Build history of the part. All positions in model axes, mm. A direction names the side the tool comes from. Coordinates: 2 decimals unless noted, no trailing zeros. Order: outer loops, then holes, each group sorted by start corner. A loop starts at its lowest first (then second) coordinate and runs counter-clockwise, first axis right, second up. Notation, with made-up numbers: M 59,-1 L 95,-1 A22 ccw 95,25 Z; hole C 84,-1 d4. An arc over 180 degrees is marked long. Write item = value, one per line. Start each with the question number.
Q1. Pin check, flat tip, straight feed: P1, Ø0.6, axis at y = 0, z = -0.5, coming from the -X side. Stop position of the tip, or through.
Q2. Drill centre lines: probe 1 along Y at (x, z) = (-0.95, -0.6); probe 2 along Y at (x, z) = (-0.15, -1.2); probe 3 along X at (y, z) = (4.75, 0.05). Where is each one in solid material? Low to high.
Q3. Band-saw the part on B-B on x = 0. Write the cut outline in (y, z).
Q4. Band-saw the part on C-C on y = 8.75. Write the cut outline in (x, z), plus the area to 3 significant figures.
Q5. 3-axis set-ups, long thin cutter, end or side, ignore diameter. For faces 1 (the face through (-1, 1.2, 0)), 2 (the face through (-1, 0, 0)): which of +Z, -Z, +X, -X, +Y, -Y reach the whole face in a straight line?
Q6. Band-saw the part on A-A on z = 0. Write the cut outline in (x, y), plus the area to 3 significant figures.
```python
from build123d import *

# Parameters (mm, degrees)
SKETCH2_R               = 1.35
BOSS_EXTRUDE1_DEPTH     = 1.2
SKETCH3_R               = 0.7
BOSS_EXTRUDE2_DEPTH     = 10
CUT_EXTRUDE1_DEPTH      = 10
CUT_EXTRUDE1_DEPTH_BACK = 10
SKETCH4_W               = 0.5
SKETCH4_H               = 0.5
FILLET1_R               = 0.2


with BuildPart() as part:
    # Sketch2 → Boss-Extrude1 (new body)
    with BuildSketch(Plane(origin=(0, 0, 0), x_dir=(1, 0, 0), z_dir=(0, 1, 0))):
        with Locations(Location((0, 0, 0), (0, 0, 270))):
            Circle(SKETCH2_R)
    extrude(amount=BOSS_EXTRUDE1_DEPTH)

    # Sketch3 → Boss-Extrude2 (add)
    with BuildSketch(Plane(origin=(0, 1.2, 0), x_dir=(1, 0, 0), z_dir=(0, 1, 0))):
        with Locations(Location((0, 0, 0), (0, 0, 270))):
            Circle(SKETCH3_R)
    extrude(amount=BOSS_EXTRUDE2_DEPTH)

    # Sketch4 → Cut-Extrude1 (cut, two sides: drawn at the far end of the back side and taken through both)
    with BuildSketch(Plane.XY.offset(-CUT_EXTRUDE1_DEPTH_BACK)):
        with Locations((0, 0.25)):
            Rectangle(SKETCH4_W, SKETCH4_H)
    extrude(amount=CUT_EXTRUDE1_DEPTH + CUT_EXTRUDE1_DEPTH_BACK, mode=Mode.SUBTRACT)

    # Fillet1
    fillet1_edges = [part.edges().sort_by_distance(p)[0] for p in [
        (-1.35, 0, 0),
        (1.35, 0, 0),
        (0, 11.2, -0.7),
    ]]
    fillet(fillet1_edges, radius=FILLET1_R)


solid = part.part
```
Recorded:
q1.P1 = -1.32
q2.probe_1 = 0 to 1.2
q2.probe_2 = 0.5 to 1.2
q2.probe_3 = -0.7 to 0.7
q3.outline = M 0.5,-1.35 L 1.2,-1.35 L 1.2,-0.7 L 11,-0.7 A0.2 ccw 11.2,-0.5 L 11.2,0.5 A0.2 ccw 11,0.7 L 1.2,0.7 L 1.2,1.35 L 0.5,1.35 Z
q4.outline = C 0,0 d1.4
q4.area = 1.54 mm2
q5.face_1 = +Y
q5.face_2 = +Z, -Z, +X, -X, -Y
q6.outline = M -1.35,0.2 A0.2 ccw -1.15,0 L -0.25,0 L -0.25,0.5 L 0.25,0.5 L 0.25,0 L 1.15,0 A0.2 ccw 1.35,0.2 L 1.35,1.2 L 0.7,1.2 L 0.7,11 A0.2 ccw 0.5,11.2 L -0.5,11.2 A0.2 ccw -0.7,11 L -0.7,1.2 L -1.35,1.2 Z
q6.area = 17.0 mm2
